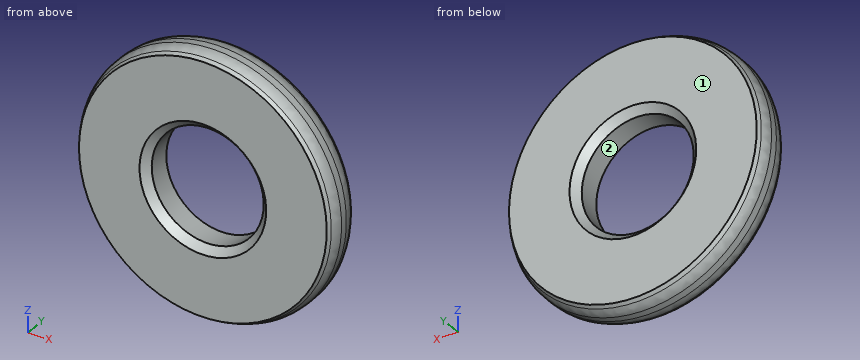
```python
from build123d import *

# Parameters (mm, degrees)
SKETCH_1_R               = 17.5
EXTRUDE_1_DEPTH          = 5
CUT_EXTRUDE_1_DEPTH      = 26.248762346
CUT_EXTRUDE_1_DEPTH_BACK = 26.248762346
SKETCH_2_R               = 7.6
CHAMFER_1_SIZE           = 1.2
CHAMFER_1_SIZE2          = 0.692820323
FILLET_1_R               = 3
CHAMFER_2_SIZE           = 1


with BuildPart() as part:
    # 스케치1 → 보스-돌출1 (new body)
    with BuildSketch(Plane(origin=(0, 0, 0), x_dir=(1, 0, 0), z_dir=(0, 1, 0))):
        with Locations(Location((0, 0, 0), (0, 0, 270))):
            Circle(SKETCH_1_R)
    extrude(amount=EXTRUDE_1_DEPTH)

    # 스케치2 → 컷-돌출1 (cut, two sides: drawn at the far end of the back side and taken through both)
    with BuildSketch(Plane(origin=(0, 5, 0), x_dir=(1, 0, 0), z_dir=(0, 1, 0)).offset(-CUT_EXTRUDE_1_DEPTH_BACK)):
        with Locations(Location((0, 0, 0), (0, 0, 270))):
            Circle(SKETCH_2_R)
    extrude(amount=CUT_EXTRUDE_1_DEPTH + CUT_EXTRUDE_1_DEPTH_BACK, mode=Mode.SUBTRACT)

    # 모따기1
    chamfer_1_edges = [part.edges().sort_by_distance(p)[0] for p in [
        (0, 0, -17.5),
        (0, 5, -17.5),
    ]]
    chamfer_1_side = [part.faces().sort_by_distance(p)[0] for p in [
        (0, 2.5, -17.5),
    ]]
    chamfer(chamfer_1_edges, length=CHAMFER_1_SIZE, length2=CHAMFER_1_SIZE2, reference=chamfer_1_side[0])

    # 필렛1
    fillet_1_edges = [part.edges().sort_by_distance(p)[0] for p in [
        (0, 1.2, -17.5),
        (0, 3.8, -17.5),
    ]]
    fillet(fillet_1_edges, radius=FILLET_1_R)

    # 모따기2
    chamfer_2_edges = [part.edges().sort_by_distance(p)[0] for p in [
        (0, 5, -7.6),
        (0, 0, -7.6),
    ]]
    chamfer(chamfer_2_edges, length=CHAMFER_2_SIZE)


solid = part.part
```
Can you work these out from the model? Positions are in its coordinate system, mm. Face numbers are marked on the shaded views. Round coordinates to 2 decimals unless told otherwise and drop trailing zeros. Answer in a Markdown table with one row per item.
1. Please list where these lines run through material, in increasing order: line 1 (X direction, y = 2.3, z = 0); line 2 (X direction, y = 4.65, z = -6.5). Write a range as from..to.
Established:
| item | result |
|---|---|
| line 1 | -17.5..-7.6, 7.6..17.5 |
| line 2 | -15.72..-5.08, 5.08..15.72 |
2. I'm going to push flat-ended pins straight in: pin 1 Ø3 at (y, z) = (4, -2) entering from +X; pin 2 Ø1 at (y, z) = (4.5, -6) entering from -X. Where does each tip first touch, or does it pass through?
Established:
| item | result |
|---|---|
| pin 1 | x = 17.48 |
| pin 2 | x = -16.32 |
3. Thinking about a two-plate mould opening in Z: for the marked faces 1 and 2, which applies, pulls with the +Z half, pulls with the -Z half, needs draft (parallel to the pull), parting line crosses it, or undercut?
Established:
| item | result |
|---|---|
| face 1 | needs draft |
| face 2 | undercut |
